Check sheet for the modelled part. Datum: model origin and axes. Units: mm. A direction names the side the tool comes from. Round coordinates to 2 decimals unless told otherwise and drop trailing zeros. Order: outer loops, then holes, each group sorted by start corner. A loop starts at its lowest first (then second) coordinate and runs counter-clockwise, first axis right, second up. Notation, with made-up numbers: (-36.5, 56.25) -> (21.5, 56.25) arc R26 ccw to (21.5, 89.25) -> close; hole circle Ø11 at (10, 31.5). An arc over 180 degrees is marked (long way). Answer in a Markdown table with one row per item. Add a question column.
1. Sectioned sample at D-D, the plane y = 35.17. Record the boundary of the cut face in (x, z) (3 decimals), then the cut area to 3 significant figures.
2. Sectioned sample at C-C, the plane z = 0.45. Count the separate pieces of the cut face and the enclosed holes in it, then the cut area to 3 significant figures.
3. Access from +Z, -Z, +X, -X, +Y, -Y to the whole of each face (thin tool, end or side, straight path). Record for faces 5 (the flat face through (-13.245, 30, 1)), 6 (the flat face through (-19.245, 10, 2)), 7 (the flat face through (-9, 0, 1)), 8 (the cylindrical face through (-32.39, 39.1, 1.52)), 9 (the flat face through (-33.245, -15, 1)).
4. Sectioned sample at A-A, the plane y = 15. Record the boundary of the cut face in (x, z) (3 decimals).
5. Depth check by flat-ended pin: P1, Ø5.5, axis at x = -27.745, y = 35.17, coming from the -Z side; P2, Ø1.5, axis at x = -8.5, z = 1, coming from the -Y side; P3, Ø1, axis at x = -11.5, z = 1.5, coming from the -Y side; P4, Ø2.5, axis at x = 0, y = -15, coming from the +Z side. Enter the tip coordinate at first touch or a pass-through.
6. Draft check along Y on faces 1 (the flat face through (-33.245, 36, 1)), 2 (the cylindrical face through (-20.1, -10.1, 1.5)), 3 (the flat face through (-26, -11, 2)), 4 (the cylindrical face through (-12.39, -0.9, 1.52)). Enter one of: +Y half, -Y half, draft (parallel to the pull), parting line (faces both ways), or undercut.
7. Material ranges on L1, parallel to X at y = -15, z = 1.6 (3 decimals); L2, parallel to Y at x = 0, z = 1.4; L3, parallel to Y at x = -26, z = 2.1, recorded low to high. Write a range as from..to.
8. Sectioned sample at B-B, the plane x = 0. Record the boundary of the cut face in (y, z), then the cut area to 3 significant figures.
```python
from build123d import *

# Parameters (mm, degrees)
SKETCH1_W           = 8
SKETCH1_H           = 40
SKETCH1_R           = 1.65
BOSS_EXTRUDE1_DEPTH = 3
SKETCH9_W           = 3
SKETCH9_H           = 20
BOSS_EXTRUDE6_DEPTH = 9.245
SKETCH10_W          = 3
SKETCH10_H          = 60
BOSS_EXTRUDE7_DEPTH = 20
SKETCH11_W          = 14
SKETCH11_H          = 42
CUT_EXTRUDE1_DEPTH  = 10
SKETCH12_R          = 1.65
CUT_EXTRUDE2_DEPTH  = 10
FILLET7_R           = 3


with BuildPart() as part:
    # Sketch1 → Boss-Extrude1 (new body)
    with BuildSketch(Plane.XY):
        Rectangle(SKETCH1_W, SKETCH1_H)
        with Locations((0, 15)):
            Circle(SKETCH1_R, mode=Mode.SUBTRACT)
        with Locations(Location((0, -15, 0), (0, 0, 180))):
            Circle(SKETCH1_R, mode=Mode.SUBTRACT)
    extrude(amount=BOSS_EXTRUDE1_DEPTH)

    # Sketch9 → Boss-Extrude6 (add)
    with BuildSketch(Plane.ZY.offset(4)):
        with Locations((1.5, 10)):
            Rectangle(SKETCH9_W, SKETCH9_H)
    extrude(amount=BOSS_EXTRUDE6_DEPTH)

    # Sketch10 → Boss-Extrude7 (add)
    with BuildSketch(Plane.ZY.offset(13.245)):
        with Locations((1.5, 10)):
            Rectangle(SKETCH10_W, SKETCH10_H)
    extrude(amount=BOSS_EXTRUDE7_DEPTH)

    # Sketch11 → Cut-Extrude1 (cut)
    with BuildSketch(Plane.XY.offset(3)):
        with Locations((-26.245, 10)):
            Rectangle(SKETCH11_W, SKETCH11_H)
    extrude(amount=-CUT_EXTRUDE1_DEPTH, mode=Mode.SUBTRACT)

    # Sketch12 → Cut-Extrude2 (cut)
    with BuildSketch(Plane.XY.offset(3)):
        with Locations((-27.745, 35.17)):
            Circle(SKETCH12_R)
        with Locations((-27.745, -15.17)):
            Circle(SKETCH12_R)
    extrude(amount=-CUT_EXTRUDE2_DEPTH, mode=Mode.SUBTRACT)

    # Fillet7
    fillet7_edges = [part.edges().sort_by_distance(p)[0] for p in [
        (-4, 0, 1.5),
        (-13.245, 0, 1.5),
        (-13.245, 20, 1.5),
        (-13.245, 40, 1.5),
        (-13.245, -20, 1.5),
        (-33.245, 40, 1.5),
        (-33.245, -20, 1.5),
        (-33.245, -11, 1.5),
        (-33.245, 31, 1.5),
        (-19.245, 31, 1.5),
        (-19.245, -11, 1.5),
        (4, -20, 1.5),
        (-4, -20, 1.5),
        (4, 20, 1.5),
    ]]
    fillet(fillet7_edges, radius=FILLET7_R)


solid = part.part
```
Answer key:
| question | item | result |
|---|---|---|
| 1 | outline | (-33.245, 0) -> (-29.395, 0) -> (-29.395, 3) -> (-33.245, 3) -> close; (-26.095, 0) -> (-13.245, 0) -> (-13.245, 3) -> (-26.095, 3) -> close |
| 1 | area | 50.1 mm² |
| 2 | separate pieces | 1 |
| 2 | enclosed holes | 4 |
| 2 | area | 1,070 mm² |
| 3 | face 5 | +Z, -Z, +X, +Y |
| 3 | face 6 | +Z, -Z, -X |
| 3 | face 7 | +Z, -Z, -Y |
| 3 | face 8 | +Z, -Z, -X, +Y |
| 3 | face 9 | +Z, -Z, -X, +Y, -Y |
| 4 | outline | (-19.245, 0) -> (-1.65, 0) -> (-1.65, 3) -> (-19.245, 3) -> close; (1.65, 0) -> (4, 0) -> (4, 3) -> (1.65, 3) -> close |
| 5 | P1 | stops at z = 0 |
| 5 | P2 | stops at y = 0 |
| 5 | P3 | stops at y = -0.57 |
| 5 | P4 | passes through |
| 6 | face 1 | draft |
| 6 | face 2 | undercut |
| 6 | face 3 | undercut |
| 6 | face 4 | -Y half |
| 7 | L1 | x = -33.245..-29.386, -26.104..-13.245, -4..-1.65, 1.65..4 |
| 7 | L2 | y = -20..-16.65, -13.35..13.35, 16.65..20 |
| 7 | L3 | y = -20..-11, 31..40 |
| 8 | outline | (-20, 0) -> (-16.65, 0) -> (-16.65, 3) -> (-20, 3) -> close; (-13.35, 0) -> (13.35, 0) -> (13.35, 3) -> (-13.35, 3) -> close; (16.65, 0) -> (20, 0) -> (20, 3) -> (16.65, 3) -> close |
| 8 | area | 100 mm² |
